For this review, take the finished solid that the model builds, in its own axes (mm). Face numbers are marked on the shaded views. Give positions to 0.01 mm unless a question says otherwise; leave off trailing zeros. Loops run counter-clockwise (first coordinate to the right, second up) from the corner with the lowest first, then second, coordinate; pieces in that order, holes last. Notation, with made-up numbers: (-6.75, 14.25) -> (21.25, 14.25) arc R13 cw to (21.25, 34.25) -> close; hole circle Ø11 at (36.25, 85.5). An arc over 180 degrees is marked (long way). One line per question, with ' | ' between items. Start each with the question number.
(1) Consider section A-A (y = 0). Write out the cut boundary in (x, z).
(2) Consider section B-B (x = 0). Write out the cut boundary in (y, z).
(3) Wall thickness on probe 1 along Y at (x, z) = (0, -0.75); probe 2 along X at (y, z) = (-1.5, -0.95); probe 3 along X at (y, z) = (0.75, -0.6): over which ranges is each line inside the solid? List them lowest first.
(4) Draft analysis for pull direction Z (two halves, no side actions). For the marked faces 1 and 2, state which applies: +Z half, -Z half, draft (parallel to the pull), parting line (faces both ways), or undercut.
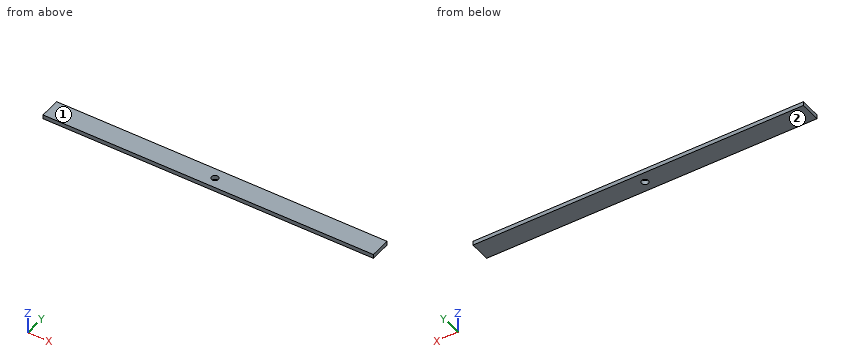
from build123d import *

# Parameters (mm, degrees)
ESBO_O1_W                                      = 160
ESBO_O1_H                                      = 10
FLANGE_BASE1_DEPTH                             = 2
BROCA_DE_ROSQUEAR_DE_CANO_PARA_TARRAXA_D_D     = 3.3
BROCA_DE_ROSQUEAR_DE_CANO_PARA_TARRAXA_D_DEPTH = 4
BROCA_DE_ROSQUEAR_DE_CANO_PARA_TARRAXA_D_TIP   = 0.991420021


# Sheet-metal steps are written as plain solids
with BuildPart() as part:
    # Esboço1 → Flange-base1 (new body)
    with BuildSketch(Plane.XY):
        Rectangle(ESBO_O1_W, ESBO_O1_H)
    extrude(amount=-FLANGE_BASE1_DEPTH)

    # Broca de rosquear de cano para tarraxa de 1/81
    with Locations(Plane(origin=(0, 0, -2), x_dir=(-1, 0, 0), z_dir=(0, 0, -1))):
        with Locations((0, 0)):
            Hole(BROCA_DE_ROSQUEAR_DE_CANO_PARA_TARRAXA_D_D / 2, depth=BROCA_DE_ROSQUEAR_DE_CANO_PARA_TARRAXA_D_DEPTH)
            with Locations((0, 0, -(BROCA_DE_ROSQUEAR_DE_CANO_PARA_TARRAXA_D_DEPTH + BROCA_DE_ROSQUEAR_DE_CANO_PARA_TARRAXA_D_TIP / 2))):  # 118° drill point
                Cone(0, BROCA_DE_ROSQUEAR_DE_CANO_PARA_TARRAXA_D_D / 2, BROCA_DE_ROSQUEAR_DE_CANO_PARA_TARRAXA_D_TIP, mode=Mode.SUBTRACT)


solid = part.part
A:
1) outline: (-80, -2) -> (-1.65, -2) -> (-1.65, 0) -> (-80, 0) -> close; (1.65, -2) -> (80, -2) -> (80, 0) -> (1.65, 0) -> close
2) outline: (-5, -2) -> (-1.65, -2) -> (-1.65, 0) -> (-5, 0) -> close; (1.65, -2) -> (5, -2) -> (5, 0) -> (1.65, 0) -> close
3) probe 1: y = -5 to -1.65, 1.65 to 5 | probe 2: x = -80 to -0.69, 0.69 to 80 | probe 3: x = -80 to -1.47, 1.47 to 80
4) face 1: +Z half | face 2: -Z half
